from build123d import *

# Parameters (mm, degrees)
F0_R     = 4.25
F1_DEPTH = 21
F2_R     = 4.25
F3_DEPTH = 21
F5_D     = 8.4
F4_R     = 4.2
F7_DEPTH = 21
F8_D     = 6.5


# Not quite as in the source:
# - a feature names something its author has since deleted; it is built from what else it names


with BuildPart() as f1:
    # F0 (on Right) → F1 (new body)
    with BuildSketch(Plane.YZ):
        Circle(F0_R)
    extrude(amount=F1_DEPTH)

    # F2 (on Right) → F3 (join)
    with BuildSketch(Plane.YZ):
        Circle(F2_R)
    extrude(amount=F3_DEPTH)

    # F5 (through all)
    with Locations(Plane(origin=(0, 0, 0), x_dir=(0, 1, 0), z_dir=(-1, 0, 0))):
        with Locations((0, 0)):
            Hole(F5_D / 2)

    # F4 (on face) → F7 (join)
    with BuildSketch(Plane.YZ):
        Circle(F4_R)
    extrude(amount=F7_DEPTH)

    # F8 (through all)
    with Locations(Plane(origin=(0, 0, 0), x_dir=(0, 1, 0), z_dir=(-1, 0, 0))):
        with Locations((0, 0)):
            Hole(F8_D / 2)


solid = f1.part
Can you work these out from the model? Positions are in its coordinate system, mm. Round coordinates to 2 decimals unless told otherwise and drop trailing zeros. Write each loop counter-clockwise with the first axis right and the second up, starting at its lowest first coordinate (ties: lowest second). Pieces come first, ordered by that corner, then holes. Notation, with made-up numbers: (-37.5, -9) - (-32.5, -9) arc R11 ccw to (-32.5, 8) - close; hole circle Ø1 at (-14.75, 88). An arc over 180 degrees is marked (long way). Write each question's results on one line, items separated by ' | '. Start each with the question number.
1) For pin 1 Ø4 at (x, y) = (16.5, -2.5) entering from -Z; pin 2 Ø5 at (x, z) = (13, 3) entering from -Y; pin 3 Ø1 at (x, y) = (9, -2.5) entering from -Z, each with a flat end and sliding along its axis, tell me the tip position at first contact or that it passes through.
2) Suppose I cut it at A-A (z = 0). List the corners of the cut face in (x, y) for me.
3) Please list where these lines run through material, in increasing order: line 1 (Z direction, x = 13, y = 0); line 2 (Y direction, x = 6.25, z = 1); line 3 (Y direction, x = 15.75, z = -0.5).
4) Suppose I cut it at C-C (x = 18.75). List the corners of the cut face in (y, z) for me.
5) We'd pull the mould along Z, two halves only. Please class faces 1 (the cylindrical face through (10.647, 2.579, 1.978)), 2 (the cylindrical face through (10.353, 2.285, 3.584)): released by +Z, released by -Z, zero draft, split by the parting line, or undercut.
Here are the results:
1) pin 1: stops at z = -4.22 | pin 2: stops at y = -4.22 | pin 3: stops at z = -3.75
2) outline: (0, -4.25) - (21, -4.25) - (21, -3.25) - (0, -3.25) - close; (0, 3.25) - (21, 3.25) - (21, 4.25) - (0, 4.25) - close
3) line 1: z = -4.25 to -3.25, 3.25 to 4.25 | line 2: y = -4.13 to -3.09, 3.09 to 4.13 | line 3: y = -4.22 to -3.21, 3.21 to 4.22
4) outline: circle Ø8.5 at (0, 0); hole circle Ø6.5 at (0, 0)
5) face 1: undercut | face 2: split by the parting line
